Part model, mm, in its own coordinate system. Face numbers are marked on the shaded views. A direction names the side the tool comes from. Give positions to 0.01 mm unless a question says otherwise; leave off trailing zeros. Order: outer loops, then holes, each group sorted by start corner. A loop starts at its lowest first (then second) coordinate and runs counter-clockwise, first axis right, second up. Notation, with made-up numbers: M 60.5,-27.75 L 94.5,-27.75 A13 ccw 94.5,-13.75 Z; hole C 14,17 d3. An arc over 180 degrees is marked long. One line per question, with ' | ' between items.
```python
from build123d import *

# Parameters (mm, degrees)
SKETCH1_R          = 3.96875
EXTRUDE1_DEPTH     = 3.96875
CUT_EXTRUDE1_DEPTH = 1.984375
SKETCH4_R          = 2.38125
EXTRUDE2_DEPTH     = 12.7
SKETCH5_R          = 2.0828
EXTRUDE3_DEPTH     = 4.7625
CHAMFER1_SIZE      = 0.47625
CUT_SWEEP1_PITCH   = 0.79375
CUT_SWEEP1_TO      = 4.7625


with BuildPart() as part:
    # Sketch1 → Extrude1 (new body)
    with BuildSketch(Plane(origin=(0, 0, 0), x_dir=(1, 0, 0), z_dir=(0, 1, 0))):
        with Locations(Location((0, 0, 0), (0, 0, 270))):
            Circle(SKETCH1_R)
    extrude(amount=EXTRUDE1_DEPTH)

    # Sketch2 → Cut-Extrude1 (cut)
    with BuildSketch(Plane(origin=(0, 3.96875, 0), x_dir=(-1, 0, 0), z_dir=(0, 1, 0))):
        Polygon((0, -1.374815329), (1.190625, -0.687407664), (1.190625, 0.687407664), (0, 1.374815329), (-1.190625, 0.687407664), (-1.190625, -0.687407664), align=None)
    extrude(amount=-CUT_EXTRUDE1_DEPTH, mode=Mode.SUBTRACT)

    # Sketch4 → Extrude2 (add)
    with BuildSketch(Plane.XZ):
        with Locations(Location((0, 0, 0), (0, 0, 90))):
            Circle(SKETCH4_R)
    extrude(amount=EXTRUDE2_DEPTH)

    # Sketch5 → Extrude3 (add)
    with BuildSketch(Plane.XZ.offset(12.7)):
        with Locations(Location((0, 0, 0), (0, 0, 90))):
            Circle(SKETCH5_R)
    extrude(amount=EXTRUDE3_DEPTH)

    # Chamfer1
    chamfer1_edges = [part.edges().sort_by_distance(p)[0] for p in [
        (0, -17.4625, -2.0828),
    ]]
    chamfer(chamfer1_edges, length=CHAMFER1_SIZE)

    # Cut-Sweep1: arcs per turn and ends read off the stored shape
    # Cut-Sweep1: the profile of Sketch13 profile screwed along a right-hand helix through 7 turns, 6 arcs to a turn; built about Z, then put on its axis
    cut_sweep1_z = Axis((0, 0, 0), (0, 0, 1))
    cut_sweep1_corners = [(2.0831, 0, -0.099045545), (2.0831, 0, -0.793923205), (1.567244252, 0, -0.49609375), (1.567244252, 0, -0.396875)]
    with BuildLine(mode=Mode.PRIVATE) as cut_sweep1_profile:
        Line(cut_sweep1_corners[0], cut_sweep1_corners[1])
        Line(cut_sweep1_corners[1], cut_sweep1_corners[2])
        Line(cut_sweep1_corners[2], cut_sweep1_corners[3])
        Line(cut_sweep1_corners[3], cut_sweep1_corners[0])
    cut_sweep1_cap = Face(cut_sweep1_profile.wire())
    cut_sweep1_turn_angles = [0, 30, 60, 90, 120, 150, 180, 210, 240, 270, 300, 330, 360]
    cut_sweep1_turn_weights = [1, 0.8660254037844387, 1, 0.8660254037844387, 1, 0.8660254037844387, 1, 0.8660254037844387, 1, 0.8660254037844387, 1, 0.8660254037844387, 1]
    cut_sweep1_turn_rails = [Edge.make_bspline([Vector(p[0], p[1], 0).rotate(cut_sweep1_z, cut_sweep1_turn_angles[k]) / cut_sweep1_turn_weights[k] + Vector(0, 0, p[2] + CUT_SWEEP1_PITCH * cut_sweep1_turn_angles[k] / 360) for k in range(13)], [0, 0, 0, 1, 1, 2, 2, 3, 3, 4, 4, 5, 5, 6, 6, 6], 2, cut_sweep1_turn_weights) for p in cut_sweep1_corners]
    cut_sweep1_turn_sides = [Face.make_surface_from_curves(cut_sweep1_turn_rails[p[0]], cut_sweep1_turn_rails[p[1]]) for p in [(0, 1), (1, 2), (2, 3), (3, 0)]]
    cut_sweep1 = Plane(origin=(0, -17.4625, 0), x_dir=(0.7071067811865438, 0, 0.7071067811865512), z_dir=(0, 1, 0)) * split(Solid(Shell([*[p.moved(Location((0, 0, CUT_SWEEP1_PITCH * i))) for i in range(7) for p in cut_sweep1_turn_sides], cut_sweep1_cap, cut_sweep1_cap.rotate(cut_sweep1_z, 2520).moved(Location((0, 0, CUT_SWEEP1_PITCH * 2520 / 360)))])), bisect_by=Plane.XY.offset(CUT_SWEEP1_TO), keep=Keep.BOTTOM, mode=Mode.PRIVATE)
    add(cut_sweep1, mode=Mode.SUBTRACT)

    # Sketch11 → Cut-Revolve7 (revolve, cut)
    with BuildSketch(Plane.XY, mode=Mode.PRIVATE) as cut_revolve7_sk:
        Polygon((3.96875, 3.806888221), (3.806888221, 3.96875), (3.96875, 3.96875), align=None)
    revolve(cut_revolve7_sk.sketch.rotate(Axis((0, 14.544175091, 0), (0, -1, 0)), 90), axis=Axis((0, 14.544175091, 0), (0, -1, 0)), mode=Mode.SUBTRACT)


solid = part.part
```
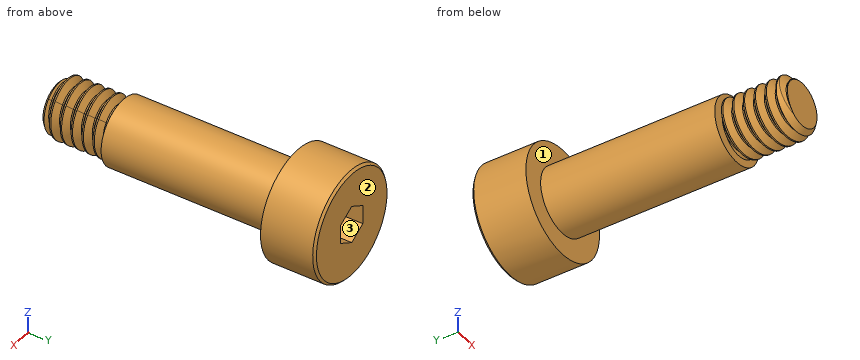
1. Tool access for the marked faces 1, 2 and 3: list every direction of +Z, -Z, +X, -X, +Y, -Y with a clear straight run to the whole face (end or side of a thin tool).
Worked out:
face 1: -Y | face 2: +Z, -Z, +X, -X, +Y | face 3: +Y
2. Slice it at A-A on y = -6. Give the cut face in (x, z), then the cut area to 3 significant figures.
Worked out:
outline: C 0,0 d4.76 | area: 17.8 mm2
3. Probe L1, parallel to Y at x = 1.5, z = -1.25; L2, parallel to Y at x = -0.25, z = -2.5; L3, parallel to Y at x = -2.25, z = -0.5. List the from-to ranges inside material, lowest first. Write a range as from..to.
Worked out:
L1: y = -16.66..-16.41, -15.86..-15.61, -15.07..-14.82, -14.28..-14.03, -13.48..-13.23, -12.7..3.97 | L2: y = 0..3.97 | L3: y = -12.7..3.97
4. Drop flat-ended pins along their axis: pin 1 (0.7 mm diameter, centred on x = -0.5, z = 0.5, fed in from +Y); pin 2 (1 mm diameter, centred on y = -13, z = 0.5, fed in from -X). Give the stop position or say it passes through.
Worked out:
pin 1: stops at y = 1.98 | pin 2: stops at x = -2.38
